Model file for the job. Use its own axes, mm. Give positions to 0.01 mm unless a question says otherwise; leave off trailing zeros. Loops run counter-clockwise (first coordinate to the right, second up) from the corner with the lowest first, then second, coordinate; pieces in that order, holes last. Notation, with made-up numbers: (77, 82.5) - (94, 82.5) arc R16 ccw to (94, 103.5) - close; hole circle Ø6 at (-14, 57). An arc over 180 degrees is marked (long way). Answer as CSV lines item,"result". Start each with the question number.
Item 1: Drill centre lines: L1, parallel to Y at x = 0, z = 42; L2, parallel to Y at x = 89, z = 33. Where is each one in solid material? Low to high. Write a range as from..to.
Item 2: Saw through at A-A on y = 0. Give the cut face in (x, z), plus the area to 3 significant figures.
Item 3: Saw through at B-B on x = -90. Give the cut face in (y, z), plus the area to 3 significant figures.
Item 4: Pin check, flat tip, straight feed: pin 1 (7 mm diameter, centred on x = -90, y = 0, fed in from -Z). Stop position of the tip, or through.
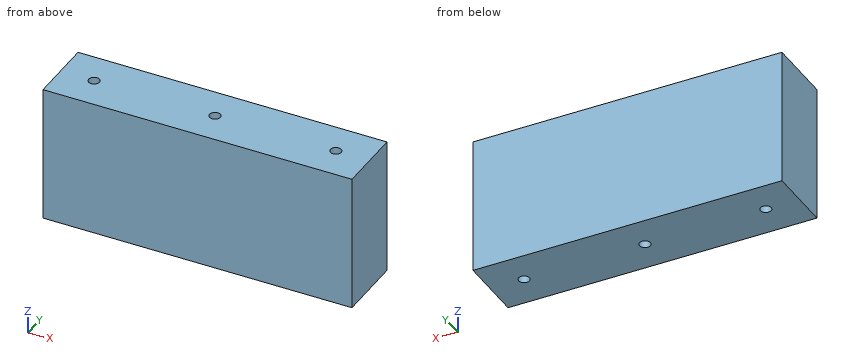
from build123d import *

# Parameters (mm, degrees)
SKETCH2_W           = 230
SKETCH2_H           = 50
BOSS_EXTRUDE1_DEPTH = 102
SKETCH3_R           = 4
CUT_EXTRUDE1_DEPTH  = 156.73695772


with BuildPart() as part:
    # Sketch2 → Boss-Extrude1 (new body)
    with BuildSketch(Plane.XY):
        Rectangle(SKETCH2_W, SKETCH2_H)
    extrude(amount=BOSS_EXTRUDE1_DEPTH)

    # Sketch3 → Cut-Extrude1 (cut, through all)
    with BuildSketch(Plane.XY.offset(102)):
        Circle(SKETCH3_R)
        with Locations((90, 0)):
            Circle(SKETCH3_R)
        with Locations((-90, 0)):
            Circle(SKETCH3_R)
    extrude(amount=-CUT_EXTRUDE1_DEPTH, mode=Mode.SUBTRACT)


solid = part.part
Responses:
1,L1,"-25..-4, 4..25"
1,L2,"-25..-3.87, 3.87..25"
2,outline,"(-115, 0) - (-94, 0) - (-94, 102) - (-115, 102) - close; (-86, 0) - (-4, 0) - (-4, 102) - (-86, 102) - close; (4, 0) - (86, 0) - (86, 102) - (4, 102) - close; (94, 0) - (115, 0) - (115, 102) - (94, 102) - close"
2,area,"21,000 mm2"
3,outline,"(-25, 0) - (-4, 0) - (-4, 102) - (-25, 102) - close; (4, 0) - (25, 0) - (25, 102) - (4, 102) - close"
3,area,"4,280 mm2"
4,pin 1,"through"
